Input: part model. Units: mm. Frame: model coordinates. A direction names the side the tool comes from. Coordinates: 2 decimals unless noted, no trailing zeros. Loops run counter-clockwise (first coordinate to the right, second up) from the corner with the lowest first, then second, coordinate; pieces in that order, holes last.
(1) Section B-B, the plane y = 20. Return loops of the section in (x, z) (1 decimal).
(2) Line query: L1, parallel to Y at x = 1, z = 2.9; L2, parallel to X at y = 15, z = 0.35; L3, parallel to Y at x = 9, z = 2.9. Output: solid intervals per line, ascending.
(3) Section C-C, the plane x = -4. Return loops of the section in (y, z) (3 decimals), then the cut area to 3 significant figures.
(4) Contact query for flat-ended pins moving along their axis: P1, Ø1.7, axis at x = -2.5, z = 1.5, coming from the -Y side; P2, Ø0.8, axis at x = 2.5, z = 1.5, coming from the -Y side; P3, Ø1, axis at y = 14.5, z = 1, coming from the +X side; P4, Ø2.5, axis at x = 0, y = 8.001, coming from the -Z side. Output: stop coordinate, or through.
(5) Set-up query: faces 1 (the face through (2, 23.406, 2)), 2 (the face through (-2, 23.406, 2)), 3 (the face through (0.59, -13.87, 1.57)). Return all of +Z, -Z, +X, -X, +Y, -Y with unobstructed straight access to the full face (end or side cutting, diameter ignored); none if empty.
(6) Section A-A, the plane z = 0.45. Return loops of the section in (x, y) (1 decimal).
(7) Mould query, pull axis X, two halves, no side actions, for faces 4 (the face through (1.623, -8.512, 1.565)), 5 (the face through (1.588, 19, 2)), 6 (the face through (-1.61, 25.91, 1.61)), 7 (the face through (-0.369, 9.662, 1.565)). Classes: released by +X, released by -X, zero draft, split by the parting line, or undercut.
Autodesk Inventor part; units mm, degrees
ref_plane "YZ Plane" through (0, 0, 0) normal (1, 0, 0) x (0, 1, 0)
ref_plane "XZ Plane" through (0, 0, 0) normal (0, 1, 0) x (-1, 0, 0)
ref_plane "XY Plane" through (0, 0, 0) normal (0, 0, 1) x (1, 0, 0)
sketch "Sketch1" plane through (0, 0, 0) normal (0, 0, 1) x (1, 0, 0)
  circle A0 centre (0, 0) radius 13.8811
  circle A1 centre (0, 0) radius 4.445
  circle A2 centre (0, 8.001) radius 1.7018
  circle A3 centre (0, -8.001) radius 1.7018
  dimension "d0" = 27.7622
  dimension "d1" = 8.89
  dimension "d2" = 16.002
  dimension "d3" = 8.001
  dimension "d4" = 3.4036
  dimension "d5" = 3.4036
extrude "Extrusion1" add sketch "Sketch1" along normal blind 3.175 contours A0 | A1
sketch "Sketch2" plane through (0, 0, 3.175) normal (0, 0, 1) x (1, 0, 0)
  line L0 (-1.5875, 12.7) -> (1.5875, 12.7)
  line L1 (1.5875, 12.7) -> (1.5875, 23.4061)
  line L2 (1.5875, 23.4061) -> (-1.5875, 23.4061)
  line L3 (-1.5875, 23.4061) -> (-1.5875, 12.7)
  circle A0 centre (0, 0) radius 13.8811
  line L4 (0, 23.4061) -> (-3.175, 23.4061)
  line L5 (-3.175, 23.4061) -> (0, 28.4861)
  line L6 (0, 23.4061) -> (0, 21.3049) construction
  line L7 (0, 23.4061) -> (3.175, 23.4061)
  line L8 (3.175, 23.4061) -> (0, 28.4861)
  point P0 (0, 12.7)
  point P1 (-1.5875, 13.79)
  point P2 (1.5875, 13.79)
  dimension "d8" = 3.175
  dimension "d9" = 9.525
  dimension "d10" = 5.08
  dimension "d11" = 3.175
  dimension "d14" = 12.7
extrude "Extrusion2" add sketch "Sketch2" against normal up to surface (3.175 mm away) contours L3 A0 L1 L0 | L3 L2 L1 A0 | L4 L5 L8 L7 L2 picked at (-0.1767, 13.0903)
properties part number "Arrow_Top"
Report:
1. outline: (-1.6, 0) - (1.6, 0) - (1.6, 3.2) - (-1.6, 3.2) - close
2. L1: y = -13.85 to -9.38, -6.62 to 6.62, 9.38 to 26.89
2. L2: x = -1.59 to 1.59
2. L3: y = -10.57 to 10.57
3. outline: (-13.292, 0) - (13.292, 0) - (13.292, 3.175) - (-13.292, 3.175) - close
3. area: 84.4 mm2
4. P1: stops at y = -13.78
4. P2: stops at y = -13.72
4. P3: stops at x = 1.59
4. P4: passes through
5. face 1: +Z, -Z, +X
5. face 2: +Z, -Z, -X
5. face 3: +Z, -Z
6. outline: (-3.2, 23.4) - (-1.6, 23.4) - (-1.6, 13.8) arc R13.9 ccw (long way) to (1.6, 13.8) - (1.6, 23.4) - (3.2, 23.4) - (0, 28.5) - close; hole circle Ø3.4 at (0, -8); hole circle Ø3.4 at (0, 8)
7. face 4: undercut
7. face 5: released by +X
7. face 6: released by -X
7. face 7: undercut
